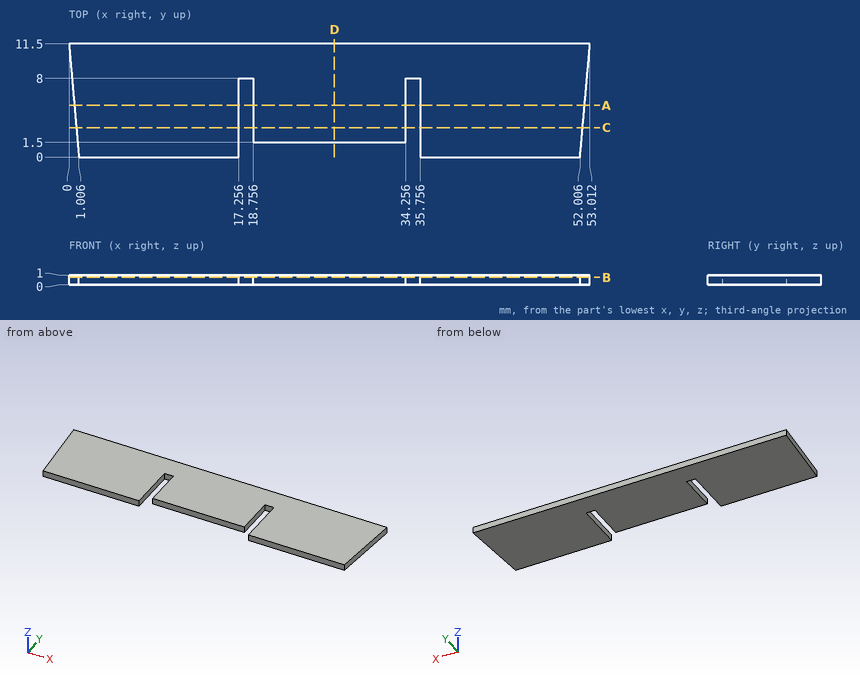
Input: dimensioned drawing with shaded views. Units: mm. Origin: part minimum x, y, z. Coordinates: 2 decimals unless noted, no trailing zeros. Order: outer loops, then holes, each group sorted by start corner. A loop starts at its lowest first (then second) coordinate and runs counter-clockwise, first axis right, second up.
(1) Material intervals for probe 1 along X at (y, z) = (7.5, 0.75); probe 2 along X at (y, z) = (6.5, 0.4) (1 decimal); probe 3 along Y at (x, z) = (29.5, 0.8), sorted ascending.
(2) Section query A-A (y = 5.25). Return the cut outline in (x, z) (1 decimal).
(3) Section query D-D (x = 27). Return the cut outline in (y, z), plus the area to 3 significant figures.
(4) Section query C-C (y = 3). Return the cut outline in (x, z).
(5) Section query B-B (z = 0.75). Return the cut outline in (x, y), plus the area to 3 significant figures.
Solution:
1. probe 1: x = 0.35 to 17.26, 18.76 to 34.26, 35.76 to 52.66
1. probe 2: x = 0.4 to 17.3, 18.8 to 34.3, 35.8 to 52.6
1. probe 3: y = 1.5 to 11.5
2. outline: (0.5, 0) - (17.3, 0) - (17.3, 1) - (0.5, 1) - close; (18.8, 0) - (34.3, 0) - (34.3, 1) - (18.8, 1) - close; (35.8, 0) - (52.5, 0) - (52.5, 1) - (35.8, 1) - close
3. outline: (1.5, 0) - (11.5, 0) - (11.5, 1) - (1.5, 1) - close
3. area: 10.0 mm2
4. outline: (0.74, 0) - (17.26, 0) - (17.26, 1) - (0.74, 1) - close; (18.76, 0) - (34.26, 0) - (34.26, 1) - (18.76, 1) - close; (35.76, 0) - (52.27, 0) - (52.27, 1) - (35.76, 1) - close
5. outline: (0, 11.5) - (1.01, 0) - (17.26, 0) - (17.26, 8) - (18.76, 8) - (18.76, 1.5) - (34.26, 1.5) - (34.26, 8) - (35.76, 8) - (35.76, 0) - (52.01, 0) - (53.01, 11.5) - close
5. area: 551 mm2
